Could you check a few things on this model? Use its own coordinates, in mm. Face numbers are marked on the shaded views. A direction names the side the tool comes from. Round coordinates to 2 decimals unless told otherwise and drop trailing zeros. Write each loop counter-clockwise with the first axis right and the second up, starting at its lowest first coordinate (ties: lowest second). Pieces come first, ordered by that corner, then holes. Notation, with made-up numbers: (78.25, 42.5) -> (100.25, 42.5) arc R19 ccw to (100.25, 73.5) -> close; hole circle Ø7 at (-36, -27.5). An arc over 180 degrees is marked (long way). Return JSON: item names as keys, results as strings.
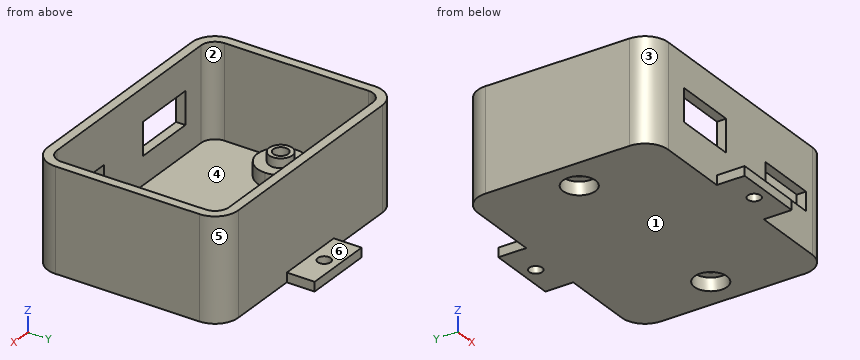
from build123d import *

# Parameters (mm, degrees)
PAD_DEPTH       = 20
THICKNESS_T     = 2
SKETCH001_W     = 15
SKETCH001_H     = 2
PAD001_DEPTH    = 6
SKETCH002_R     = 1.4
POCKET_DEPTH    = 2.001
SKETCH003_W     = 15
SKETCH003_H     = 2
PAD002_DEPTH    = 6
SKETCH004_R     = 1.4
POCKET001_DEPTH = 22.001
SKETCH005_R     = 2.5
PAD003_DEPTH    = 7
SKETCH006_R     = 5
PAD004_DEPTH    = 5
SKETCH007_R     = 1.6
POCKET002_DEPTH = 22.001
SKETCH008_R     = 3.5
POCKET003_DEPTH = 2.8
SKETCH009_W     = 13.5
SKETCH009_H     = 7
SKETCH009_W_2   = 13
SKETCH009_H_2   = 4
POCKET004_DEPTH = 2


with BuildPart() as part:
    # Sketch → Pad (new body)
    with BuildSketch(Plane.XY):
        with BuildLine():
            Line((0, 37), (46, 37))
            ThreePointArc((49, 34), (48.1213203436, 36.1213203436), (46, 37))
            Line((49, 34), (49, 3))
            ThreePointArc((46, 0), (48.1213203436, 0.8786796564), (49, 3))
            Line((46, 0), (0, 0))
            ThreePointArc((-3, 3), (-2.1213203436, 0.8786796564), (0, 0))
            Line((-3, 3), (-3, 34))
            ThreePointArc((0, 37), (-2.1213203436, 36.1213203436), (-3, 34))
        make_face()
    extrude(amount=PAD_DEPTH)

    # Thickness
    thickness_openings = [part.faces().sort_by_distance(p)[0] for p in [
        (23, 18.5, 20),
    ]]
    offset(amount=THICKNESS_T, openings=thickness_openings, kind=Kind.INTERSECTION)

    # Sketch001 → Pad001 (new body)
    with BuildSketch(Plane(origin=(0, 39, 0), x_dir=(-1, 0, 0), z_dir=(0, 1, 0))):
        with Locations((-23, -1)):
            Rectangle(SKETCH001_W, SKETCH001_H)
    extrude(amount=PAD001_DEPTH)

    # Sketch002 → Pocket (cut, through all)
    with BuildSketch(Plane.XY):
        with Locations((23, 42)):
            Circle(SKETCH002_R)
    extrude(amount=-POCKET_DEPTH, mode=Mode.SUBTRACT)

    # Sketch003 → Pad002 (new body)
    with BuildSketch(Plane.XZ.offset(2)):
        with Locations((23, -1)):
            Rectangle(SKETCH003_W, SKETCH003_H)
    extrude(amount=PAD002_DEPTH)

    # Sketch004 → Pocket001 (cut, through all)
    with BuildSketch(Plane(origin=(0, 0, -2), x_dir=(1, 0, 0), z_dir=(0, 0, -1))):
        with Locations((23, 5)):
            Circle(SKETCH004_R)
    extrude(amount=-POCKET001_DEPTH, mode=Mode.SUBTRACT)

    # Sketch005 → Pad003 (new body)
    with BuildSketch(Plane(origin=(0, 0, -2), x_dir=(1, 0, 0), z_dir=(0, 0, -1))):
        with Locations((2, -18.5)):
            Circle(SKETCH005_R)
        with Locations((44, -18.5)):
            Circle(SKETCH005_R)
    extrude(amount=-PAD003_DEPTH)

    # Sketch006 → Pad004 (new body)
    with BuildSketch(Plane(origin=(0, 0, -2), x_dir=(1, 0, 0), z_dir=(0, 0, -1))):
        with Locations((2, -18.5)):
            Circle(SKETCH006_R)
        with Locations((44, -18.5)):
            Circle(SKETCH006_R)
    extrude(amount=-PAD004_DEPTH)

    # Sketch007 → Pocket002 (cut, through all)
    with BuildSketch(Plane(origin=(0, 0, -2), x_dir=(1, 0, 0), z_dir=(0, 0, -1))):
        with Locations((2, -18.5)):
            Circle(SKETCH007_R)
        with Locations((44, -18.5)):
            Circle(SKETCH007_R)
    extrude(amount=-POCKET002_DEPTH, mode=Mode.SUBTRACT)

    # Sketch008 → Pocket003 (cut)
    with BuildSketch(Plane(origin=(0, 0, -2), x_dir=(1, 0, 0), z_dir=(0, 0, -1))):
        with Locations((2, -18.5)):
            Circle(SKETCH008_R)
        with Locations((44, -18.5)):
            Circle(SKETCH008_R)
    extrude(amount=-POCKET003_DEPTH, mode=Mode.SUBTRACT)

    # Sketch009 → Pocket004 (cut)
    with BuildSketch(Plane.XZ.offset(2)):
        with Locations((11.75, 9.5)):
            Rectangle(SKETCH009_W, SKETCH009_H)
        with Locations((37.5, 8)):
            Rectangle(SKETCH009_W_2, SKETCH009_H_2)
    extrude(amount=-POCKET004_DEPTH, mode=Mode.SUBTRACT)


solid = part.part
1) If I drill on probe 1 along X at (y, z) = (18.5, 4.1); probe 2 along Y at (x, z) = (44, 2.9); probe 3 along X at (y, z) = (18.5, -0.15), over which ranges is the centre line in solid material (lowest first)? Write a range as [from, to].
Return value:
{"probe 1": "[-5, -3], [-0.5, 0.4], [3.6, 4.5], [41.5, 42.4], [45.6, 46.5], [49, 51]", "probe 2": "[-2, 0], [13.5, 16.9], [20.1, 23.5], [37, 39]", "probe 3": "[-5, -1.5], [5.5, 40.5], [47.5, 51]"}
2) I want a section at A-A, the plane z = 3.75. Please give me the cut outline in (x, y), and give its area (3 significant figures).
Return value:
{"outline": "(-5, 3) arc R5 ccw to (0, -2) -> (46, -2) arc R5 ccw to (51, 3) -> (51, 34) arc R5 ccw to (46, 39) -> (0, 39) arc R5 ccw to (-5, 34) -> close; circle Ø5 at (2, 18.5); circle Ø5 at (44, 18.5); hole (-3, 3) arc R3 ccw to (0, 0) -> (46, 0) arc R3 ccw to (49, 3) -> (49, 34) arc R3 ccw to (46, 37) -> (0, 37) arc R3 ccw to (-3, 34) -> close; hole circle Ø3.2 at (2, 18.5); hole circle Ø3.2 at (44, 18.5)", "area": "381 mm²"}
3) I want a section at B-B, the plane y = 42. Please give me the cut outline in (x, z), and give its area (3 significant figures).
Return value:
{"outline": "(15.5, -2) -> (21.6, -2) -> (21.6, 0) -> (15.5, 0) -> close; (24.4, -2) -> (30.5, -2) -> (30.5, 0) -> (24.4, 0) -> close", "area": "24.4 mm²"}
4) For the marked faces 1 and 2, which set-ups out of +Z, -Z, +X, -X, +Y, -Y let a thin tool reach every point of the face, with its end or its side?
Return value:
{"face 1": "-Z, +X, -X, +Y, -Y", "face 2": "+Z"}
5) Will these pins go through, and if not, where does the flat tip stop? pin 1 Ø10 at (x, z) = (27, 7) entering from -Y; pin 2 Ø2 at (x, z) = (1, 8.5) entering from +Y; pin 3 Ø2 at (y, z) = (-5, -1.5) entering from +X; pin 4 Ø1.9 at (x, y) = (2, 18.5) entering from +Z.
Return value:
{"pin 1": "y = -2", "pin 2": "y = 39", "pin 3": "x = 30.5", "pin 4": "through"}
6) I want a section at D-D, the plane x = 23. Please give me the cut outline in (y, z).
Return value:
{"outline": "(-8, -2) -> (-6.4, -2) -> (-6.4, 0) -> (-8, 0) -> close; (-3.6, -2) -> (40.6, -2) -> (40.6, 0) -> (39, 0) -> (39, 20) -> (37, 20) -> (37, 0) -> (0, 0) -> (0, 20) -> (-2, 20) -> (-2, 0) -> (-3.6, 0) -> close; (43.4, -2) -> (45, -2) -> (45, 0) -> (43.4, 0) -> close"}
7) I want a section at C-C, the plane x = 2. Please give me the cut outline in (y, z), and give its area (3 significant figures).
Return value:
{"outline": "(-2, -2) -> (15, -2) -> (15, 0.8) -> (16.9, 0.8) -> (16.9, 5) -> (16, 5) -> (16, 3) -> (13.5, 3) -> (13.5, 0) -> (0, 0) -> (0, 20) -> (-2, 20) -> close; (20.1, 0.8) -> (22, 0.8) -> (22, -2) -> (39, -2) -> (39, 20) -> (37, 20) -> (37, 0) -> (23.5, 0) -> (23.5, 3) -> (21, 3) -> (21, 5) -> (20.1, 5) -> close", "area": "169 mm²"}
8) Thinking about a two-plate mould opening in Y: for the marked faces 3, 4, 5 and 6, which applies, pulls with the +Y half, pulls with the -Y half, needs draft (parallel to the pull), parting line crosses it, or undercut?
Return value:
{"face 3": "pulls with the -Y half", "face 4": "undercut", "face 5": "pulls with the +Y half", "face 6": "needs draft"}
